Job drawing, mm, ordinate dimensions from the low corner. One solid piece. A direction names the side the tool comes from. Round coordinates to 2 decimals unless told otherwise and drop trailing zeros. Order: outer loops, then holes, each group sorted by start corner. A loop starts at its lowest first (then second) coordinate and runs counter-clockwise, first axis right, second up. Notation, with made-up numbers: (-40, 75) -> (9, 75) arc R16 ccw to (9, 88) -> close; hole circle Ø11 at (32.25, -28). An arc over 180 degrees is marked (long way). Answer as a JSON object with one key per item and string values. Group by question number.
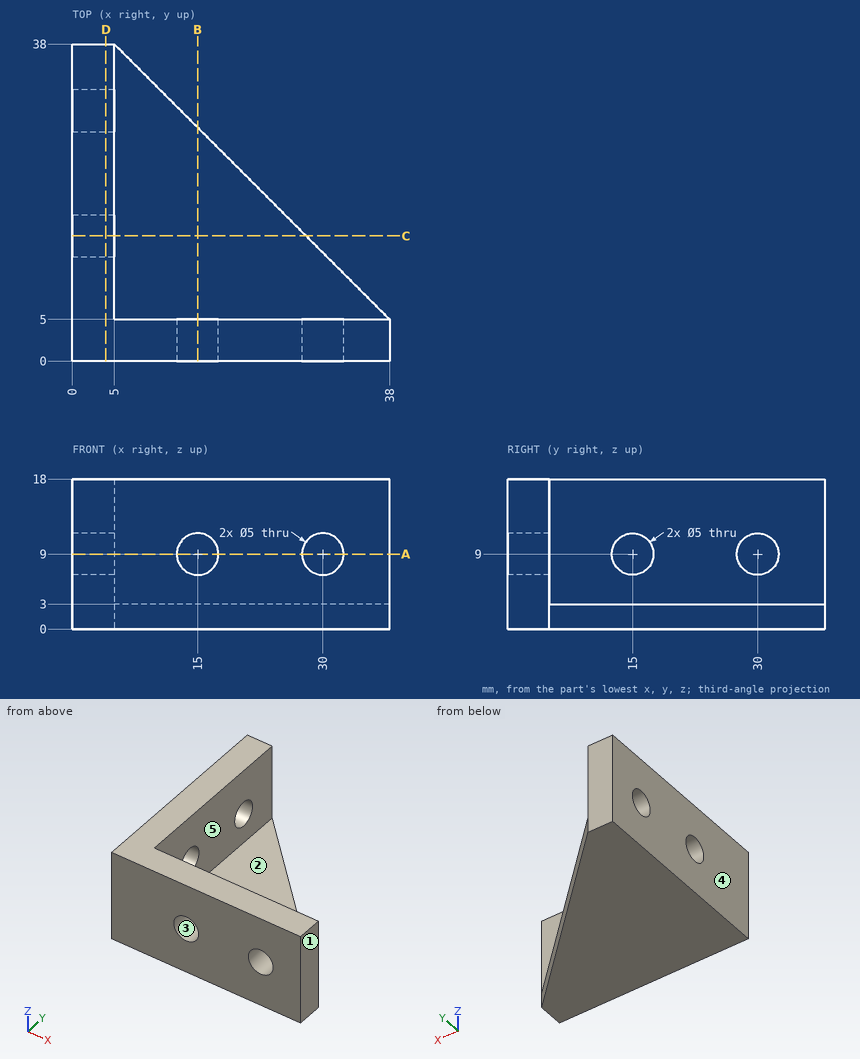
Q1. Two-plate mould, pull along X, no slides. Class the marked faces 1, 2 and 3: +X half, -X half, draft (parallel to the pull), parting line (faces both ways), or undercut.
Q2. Band-saw the part on D-D (x = 4). List the corners of the cut face in (y, z).
Q3. Band-saw the part on A-A (z = 9). List the corners of the cut face in (x, y).
Q4. Drop flat-ended pins along their axis: pin 1 Ø4 at (y, z) = (26, 4.5) entering from -X; pin 2 Ø6 at (x, z) = (15, 9) entering from +Y; pin 3 Ø8 at (y, z) = (18, 2) entering from +X; pin 4 Ø5 at (x, z) = (20.5, 2) entering from +Y. Give the stop position or say it passes through.
Q5. Which spindle directions (+Z, -Z, +X, -X, +Y, -Y) get a long thin tool onto all of the face, cutting with end or side? Do the marked faces 4 and 5. Say none if no direction does.
Q6. Band-saw the part on B-B (x = 15). List the corners of the cut face in (y, z), plus the area to 3 significant figures.
Q7. Wall check: line 1 (Z direction, x = 3.3, y = 15); line 2 (X direction, y = 18.5, z = 6.5); line 3 (Z direction, x = 9, y = 8). Give the ranges that are in metal, low to high. Write a range as [from, to].
Completed:
{
 "1": {"face 1": "+X half", "face 2": "draft", "face 3": "undercut"},
 "2": {"outline": "(0, 0) -> (38, 0) -> (38, 18) -> (0, 18) -> close; hole circle Ø5 at (15, 9); hole circle Ø5 at (30, 9)"},
 "3": {"outline": "(0, 0) -> (12.5, 0) -> (12.5, 5) -> (5, 5) -> (5, 12.5) -> (0, 12.5) -> close; (0, 17.5) -> (5, 17.5) -> (5, 27.5) -> (0, 27.5) -> close; (0, 32.5) -> (5, 32.5) -> (5, 38) -> (0, 38) -> close; (17.5, 0) -> (27.5, 0) -> (27.5, 5) -> (17.5, 5) -> close; (32.5, 0) -> (38, 0) -> (38, 5) -> (32.5, 5) -> close"},
 "4": {"pin 1": "x = 0", "pin 2": "y = 5", "pin 3": "x = 29", "pin 4": "y = 25"},
 "5": {"face 4": "+Z, -Z, -X, +Y, -Y", "face 5": "+Z, +X, +Y"},
 "6": {"outline": "(0, 0) -> (28, 0) -> (28, 3) -> (5, 3) -> (5, 6.5) -> (0, 6.5) -> close; (0, 11.5) -> (5, 11.5) -> (5, 18) -> (0, 18) -> close", "area": "134 mm2"},
 "7": {"line 1": "[0, 6.5], [11.5, 18]", "line 2": "[0, 5]", "line 3": "[0, 3]"}
}
